Can you work these out from the model? Positions are in its coordinate system, mm. A direction names the side the tool comes from. Give positions to 0.01 mm unless a question says otherwise; leave off trailing zeros. Loops run counter-clockwise (first coordinate to the right, second up) from the corner with the lowest first, then second, coordinate; pieces in that order, holes last. Notation, with made-up numbers: M 76,55.25 L 109,55.25 A26 ccw 109,80.25 Z; hole C 75,-29.5 d7. An arc over 180 degrees is marked long. Answer as a JSON object with one key per item and string values.
Autodesk Inventor part; units mm, degrees
ref_plane "YZ Plane" through (0, 0, 0) normal (1, 0, 0) x (0, 1, 0)
ref_plane "XZ Plane" through (0, 0, 0) normal (0, 1, 0) x (-1, 0, 0)
ref_plane "XY Plane" through (0, 0, 0) normal (0, 0, 1) x (1, 0, 0)
sketch "Skizze12" plane through (0, 0, 0) normal (0, 1, 0) x (-1, 0, 0)
  line L0 (0, 0) -> (200, 0)
  line L1 (200, 0) -> (200, -300)
  dimension "d28" = 200
  dimension "d29" = 300
sketch "Skizze13" plane through (0, 0, 0) normal (1, 0, 0) x (0, 1, 0)
  circle A0 centre (0, 0) radius 10
  circle A1 centre (0, 0) radius 7.5
  dimension "d30" = 20
  dimension "d31" = 15
sweep "Sweeping2" add profiles "Skizze13" path "Skizze12"
sketch "Skizze14" plane through (0, 0, 0) normal (0, 1, 0) x (-1, 0, 0)
  line L0 (0, 0) -> (10, 0)
  circle A0 centre (10, 0) radius 4
  dimension "d34" = 10
  dimension "d35" = 8
extrude "Extrusion3" cut sketch "Skizze14" along normal through all both and the other way through all
fillet "Rundung1" radius 2 2 edges at (-200, -10, -300) (-200, -7.5, -300)
properties part number "Steuerhebel" material "Edelstahl"
1) Suppose I cut it at C-C, the plane x = -10. Write out the boundary of the cut face in (y, z), and give its area (3 significant figures).
Answer list:
{"outline": "M -9.17,-4 A10 ccw 9.17,-4 L 6.34,-4 A7.5 cw -6.34,-4 Z; M -9.17,4 L -6.34,4 A7.5 cw 6.34,4 L 9.17,4 A10 ccw Z", "area": "95.9 mm^2"}
2) Suppose I cut it at D-D, the plane x = -200. Write out the boundary of the cut face in (y, z), and give its area (3 significant figures).
Answer list:
{"outline": "M -10,-298 A2 ccw -8,-300 A2 ccw -7.5,-298.68 L -7.5,0 A7.5 cw 7.5,0 L 7.5,-298.68 A2 ccw 8,-300 A2 ccw 10,-298 L 10,0 A10 ccw -10,0 Z", "area": "1,570 mm^2"}
3) Suppose I cut it at B-B, the plane y = 0. Write out the boundary of the cut face in (x, z), and give its area (3 significant figures).
Answer list:
{"outline": "M -210,-298 A2 ccw -208,-300 A2 ccw -207.5,-298.68 L -207.5,7.5 L 0,7.5 L 0,10 L -210,10 Z; M -192.5,-298.68 A2 ccw -192,-300 A2 ccw -190,-298 L -190,-10 L 0,-10 L 0,-7.5 L -192.5,-7.5 Z", "area": "2,500 mm^2"}
4) For faces 1 (the cylindrical face through (-9.479, 8.146, -3.966)), 2 (the cylindrical face through (-105.2, -1.63, 7.32)), which set-ups out of +Z, -Z, +X, -X, +Y, -Y let a thin tool reach every point of the face, with its end or its side?
Answer list:
{"face 1": "+Y, -Y", "face 2": "+X"}
5) Will these pins go through, and if not, where does the flat tip stop? pin 1 Ø10.5 at (x, z) = (-10, 0) entering from -Y; pin 2 Ø1 at (x, y) = (-165, -3.5) entering from +Z; pin 3 Ø4 at (x, y) = (-124.5, 6) entering from +Z; pin 4 Ø12 at (x, y) = (-45.5, 5) entering from -Z.
Answer list:
{"pin 1": "y = -10", "pin 2": "z = 9.54", "pin 3": "z = 9.17", "pin 4": "z = -10"}
6) If we mould it in two halves opening along Y, with no side actions, what happens to faces 3 (the flat face through (0, -7, 4)), 4 (the cylindrical face through (-209.76, -2.17, -146.16)), 5 (the cylindrical face through (-192.564, -0.976, -147.732))? For each: +Y half, -Y half, draft (parallel to the pull), parting line (faces both ways), or undercut.
Answer list:
{"face 3": "draft", "face 4": "parting line", "face 5": "undercut"}
7) Suppose I cut it at A-A, the plane z = 0. Write out the boundary of the cut face in (x, y), and give its area (3 significant figures).
Answer list:
{"outline": "M -200,-10 L -14,-10 L -14,-7.5 L -200,-7.5 A7.5 cw -200,7.5 L -14,7.5 L -14,10 L -200,10 A10 ccw Z; M -6,-10 L 0,-10 L 0,-7.5 L -6,-7.5 Z; M -6,7.5 L 0,7.5 L 0,10 L -6,10 Z", "area": "1,030 mm^2"}
8) Please list where these lines run through material, in increasing order: line 1 along Y through (x, z) = (-75, 0); line 2 along X through (y, z) = (0, -106.5). Write a range as from..to.
Answer list:
{"line 1": "-10..-7.5, 7.5..10", "line 2": "-210..-207.5, -192.5..-190"}
